```python
from build123d import *

# Parameters (mm, degrees)
BASE_DEPTH          = 3
SKETCH2_R           = 1.5
CUT_EXTRUDE1_DEPTH  = 36.920050111
CUT_EXTRUDE2_DEPTH  = 36.920050111
SKETCH6_R           = 3
CUT_EXTRUDE3_DEPTH  = 1.5
CHAMFER2_SIZE       = 0.5
BOSS_EXTRUDE1_START = -2.5
BOSS_EXTRUDE1_DEPTH = 2.5
CUT_EXTRUDE4_START  = -2.5
CUT_EXTRUDE4_DEPTH  = 2.5


# Read off the part's stored shape, not the designer's step: Cut-Extrude4
with BuildPart() as part:
    # Sketch1 → Base (new body)
    with BuildSketch(Plane.XY):
        with BuildLine():
            Line((11, -32.5), (-11, -32.5))
            ThreePointArc((-11, -32.5), (-13.828427125, -31.328427125), (-15, -28.5))
            Line((-15, -28.5), (-15, 28.5))
            ThreePointArc((-15, 28.5), (-13.828427125, 31.328427125), (-11, 32.5))
            Line((-11, 32.5), (11, 32.5))
            ThreePointArc((11, 32.5), (13.828427125, 31.328427125), (15, 28.5))
            Line((15, 28.5), (15, -28.5))
            ThreePointArc((15, -28.5), (13.828427125, -31.328427125), (11, -32.5))
        make_face()
    extrude(amount=BASE_DEPTH)

    # Sketch2 → Cut-Extrude1 (cut, through all)
    with BuildSketch(Plane.XY.offset(3)):
        with Locations((-11, 28.5)):
            Circle(SKETCH2_R)
        with Locations((-11, -28.5)):
            Circle(SKETCH2_R)
        with Locations((11, -28.5)):
            Circle(SKETCH2_R)
        with Locations((11, 28.5)):
            Circle(SKETCH2_R)
    extrude(amount=-CUT_EXTRUDE1_DEPTH, mode=Mode.SUBTRACT)

    # Sketch3 → Cut-Extrude2 (cut, through all)
    with BuildSketch(Plane.XY.offset(3)):
        with BuildLine():
            Line((6.5, 28.5), (6.5, 30.5))
            Line((6.5, 30.5), (-6.5, 30.5))
            Line((-6.5, 30.5), (-6.5, 28.5))
            ThreePointArc((-6.5, 28.5), (-7.818019485, 25.318019485), (-11, 24))
            Line((-11, 24), (-13, 24))
            Line((-13, 24), (-13, -24))
            Line((-13, -24), (-11, -24))
            ThreePointArc((-11, -24), (-7.818019485, -25.318019485), (-6.5, -28.5))
            Line((-6.5, -28.5), (-6.5, -30.5))
            Line((-6.5, -30.5), (6.5, -30.5))
            Line((6.5, -30.5), (6.5, -28.5))
            ThreePointArc((6.5, -28.5), (7.818019485, -25.318019485), (11, -24))
            Line((11, -24), (13, -24))
            Line((13, -24), (13, 24))
            Line((13, 24), (11, 24))
            ThreePointArc((11, 24), (7.818019485, 25.318019485), (6.5, 28.5))
        make_face()
    extrude(amount=-CUT_EXTRUDE2_DEPTH, mode=Mode.SUBTRACT)

    # Sketch6 → Cut-Extrude3 (cut)
    with BuildSketch(Plane.XY.offset(3)):
        with Locations((-11, -28.5)):
            Circle(SKETCH6_R)
        with Locations((11, -28.5)):
            Circle(SKETCH6_R)
        with Locations((11, 28.5)):
            Circle(SKETCH6_R)
        with Locations((-11, 28.5)):
            Circle(SKETCH6_R)
    extrude(amount=-CUT_EXTRUDE3_DEPTH, mode=Mode.SUBTRACT)

    # Chamfer2
    chamfer2_edges = [part.edges().sort_by_distance(p)[0] for p in [
        (7.818019485, 25.318019485, 3),
        (13, 0, 3),
        (7.818019485, -25.318019485, 3),
        (-7.818019485, -25.318019485, 3),
        (-13, 0, 3),
        (-7.818019485, 25.318019485, 3),
        (0, -32.5, 3),
        (-13.828427125, -31.328427125, 3),
        (-15, 0, 3),
        (-13.828427125, 31.328427125, 3),
        (0, 32.5, 3),
        (13.828427125, 31.328427125, 3),
        (15, 0, 3),
        (13.828427125, -31.328427125, 3),
        (-14, -28.5, 3),
        (-14, 28.5, 3),
        (8, 28.5, 3),
        (8, -28.5, 3),
        (0, -30.5, 3),
        (0, 30.5, 3),
        (12, 24, 3),
        (6.5, 29.5, 3),
        (-6.5, 29.5, 3),
        (-12, 24, 3),
        (-12, -24, 3),
        (-6.5, -29.5, 3),
        (6.5, -29.5, 3),
        (12, -24, 3),
    ]]
    chamfer(chamfer2_edges, length=CHAMFER2_SIZE - 0.0001)  # a hair under: the kernel refuses the full size

    # Sketch9 → Boss-Extrude1 (add)
    with BuildSketch(Plane(origin=(0, 0, 0), x_dir=(-1, 0, 0), z_dir=(0, 0, -1)).offset(BOSS_EXTRUDE1_START)):
        with BuildLine():
            ThreePointArc((-6.5, -28.5), (-7.818019485, -25.318019485), (-11, -24))
            Line((-11, -24), (-13, -24))
            Line((-13, -24), (-13, 24))
            Line((-13, 24), (-11, 24))
            ThreePointArc((-11, 24), (-7.818019485, 25.318019485), (-6.5, 28.5))
            Line((-6.5, 28.5), (-6.5, 30.5))
            Line((-6.5, 30.5), (6.5, 30.5))
            Line((6.5, 30.5), (6.5, 28.5))
            ThreePointArc((6.5, 28.5), (7.818019485, 25.318019485), (11, 24))
            Line((11, 24), (13, 24))
            Line((13, 24), (13, -24))
            Line((13, -24), (11, -24))
            ThreePointArc((11, -24), (7.818019485, -25.318019485), (6.5, -28.5))
            Line((6.5, -28.5), (6.5, -30.5))
            Line((6.5, -30.5), (-6.5, -30.5))
            Line((-6.5, -30.5), (-6.5, -28.5))
        make_face()
    extrude(amount=BOSS_EXTRUDE1_DEPTH)

    # Cut-Extrude4 outline → Cut-Extrude4 (cut)
    with BuildSketch(Plane(origin=(0, 0, 0), x_dir=(-1, 0, 0), z_dir=(0, 0, -1)).offset(CUT_EXTRUDE4_START)):
        with BuildLine():
            ThreePointArc((11.25, -6.35), (12.75, -4.85), (11.25, -3.35))
            Line((11.25, -3.35), (-11.25, -3.35))
            ThreePointArc((-11.25, -3.35), (-12.75, -4.85), (-11.25, -6.35))
            Line((-11.25, -6.35), (11.25, -6.35))
        make_face()
        with BuildLine():
            ThreePointArc((11.25, 17.9), (12.75, 19.4), (11.25, 20.9))
            Line((11.25, 20.9), (-11.25, 20.9))
            ThreePointArc((-11.25, 20.9), (-12.75, 19.4), (-11.25, 17.9))
            Line((-11.25, 17.9), (11.25, 17.9))
        make_face()
        with BuildLine():
            Line((-11, 24), (-12.729019946, 24))
            ThreePointArc((-12.729019946, 24), (-12.218245837, 23.104356076), (-11.25, 22.75))
            Line((-11.25, 22.75), (11.25, 22.75))
            ThreePointArc((11.25, 22.75), (12.218245837, 23.104356076), (12.729019946, 24))
            Line((12.729019946, 24), (11, 24))
            ThreePointArc((11, 24), (9.015686517, 24.461126395), (7.438048288, 25.75))
            Line((7.438048288, 25.75), (-7.438048288, 25.75))
            ThreePointArc((-7.438048288, 25.75), (-9.015686517, 24.461126395), (-11, 24))
        make_face()
        with BuildLine():
            ThreePointArc((-6.5, 28.5), (-6.522787311, 28.047709671), (-6.590918463, 27.6))
            Line((-6.590918463, 27.6), (6.590918463, 27.6))
            ThreePointArc((6.590918463, 27.6), (6.522787311, 28.047709671), (6.5, 28.5))
            Line((6.5, 28.5), (6.5, 30.5))
            Line((6.5, 30.5), (-6.5, 30.5))
            Line((-6.5, 30.5), (-6.5, 28.5))
        make_face()
        with BuildLine():
            Line((-6.5, -28.5), (-6.5, -30.5))
            Line((-6.5, -30.5), (6.5, -30.5))
            Line((6.5, -30.5), (6.5, -28.5))
            ThreePointArc((6.5, -28.5), (6.522787311, -28.047709671), (6.590918463, -27.6))
            Line((6.590918463, -27.6), (-6.590918463, -27.6))
            ThreePointArc((-6.590918463, -27.6), (-6.522787311, -28.047709671), (-6.5, -28.5))
        make_face()
        with BuildLine():
            Line((-11.25, -1.5), (11.25, -1.5))
            ThreePointArc((11.25, -1.5), (12.75, 0), (11.25, 1.5))
            Line((11.25, 1.5), (-11.25, 1.5))
            ThreePointArc((-11.25, 1.5), (-12.75, 0), (-11.25, -1.5))
        make_face()
        with BuildLine():
            ThreePointArc((11.25, -11.2), (12.75, -9.7), (11.25, -8.2))
            Line((11.25, -8.2), (-11.25, -8.2))
            ThreePointArc((-11.25, -8.2), (-12.75, -9.7), (-11.25, -11.2))
            Line((-11.25, -11.2), (11.25, -11.2))
        make_face()
        with BuildLine():
            ThreePointArc((11.25, -16.05), (12.75, -14.55), (11.25, -13.05))
            Line((11.25, -13.05), (-11.25, -13.05))
            ThreePointArc((-11.25, -13.05), (-12.75, -14.55), (-11.25, -16.05))
            Line((-11.25, -16.05), (11.25, -16.05))
        make_face()
        with BuildLine():
            ThreePointArc((11.25, -20.9), (12.75, -19.4), (11.25, -17.9))
            Line((11.25, -17.9), (-11.25, -17.9))
            ThreePointArc((-11.25, -17.9), (-12.75, -19.4), (-11.25, -20.9))
            Line((-11.25, -20.9), (11.25, -20.9))
        make_face()
        with BuildLine():
            ThreePointArc((12.729019946, -24), (12.218245837, -23.104356076), (11.25, -22.75))
            Line((11.25, -22.75), (-11.25, -22.75))
            ThreePointArc((-11.25, -22.75), (-12.218245837, -23.104356076), (-12.729019946, -24))
            Line((-12.729019946, -24), (-11, -24))
            ThreePointArc((-11, -24), (-9.015686517, -24.461126395), (-7.438048288, -25.75))
            Line((-7.438048288, -25.75), (7.438048288, -25.75))
            ThreePointArc((7.438048288, -25.75), (9.015686517, -24.461126395), (11, -24))
            Line((11, -24), (12.729019946, -24))
        make_face()
        with BuildLine():
            ThreePointArc((11.25, 3.35), (12.75, 4.85), (11.25, 6.35))
            Line((11.25, 6.35), (-11.25, 6.35))
            ThreePointArc((-11.25, 6.35), (-12.75, 4.85), (-11.25, 3.35))
            Line((-11.25, 3.35), (11.25, 3.35))
        make_face()
        with BuildLine():
            ThreePointArc((11.25, 8.2), (12.75, 9.7), (11.25, 11.2))
            Line((11.25, 11.2), (-11.25, 11.2))
            ThreePointArc((-11.25, 11.2), (-12.75, 9.7), (-11.25, 8.2))
            Line((-11.25, 8.2), (11.25, 8.2))
        make_face()
        with BuildLine():
            ThreePointArc((11.25, 13.05), (12.75, 14.55), (11.25, 16.05))
            Line((11.25, 16.05), (-11.25, 16.05))
            ThreePointArc((-11.25, 16.05), (-12.75, 14.55), (-11.25, 13.05))
            Line((-11.25, 13.05), (11.25, 13.05))
        make_face()
    extrude(amount=CUT_EXTRUDE4_DEPTH, mode=Mode.SUBTRACT)


solid = part.part
```
Geometry check sheet. Reference: the model listing, model coordinates, mm. A direction names the side the tool comes from. Give positions to 0.01 mm unless a question says otherwise; leave off trailing zeros. Order: outer loops, then holes, each group sorted by start corner. A loop starts at its lowest first (then second) coordinate and runs counter-clockwise, first axis right, second up. Notation, with made-up numbers: (-30, 86) - (12, 86) arc R7 ccw to (12, 91) - close; hole circle Ø5 at (-23, 6). An arc over 180 degrees is marked (long way). Write item = value, one per line. Start each with the question number.
1) Draft check along Y on faces 1 (the cylindrical face through (11, 30, 1)), 2 (the flat face through (-15, 0, 1)), 3 (the flat face through (0, -1.5, 1)), 4 (the cylindrical face through (-13.859, 31.297, 1.233)). Enter one of: released by +Y, released by -Y, zero draft, split by the parting line, or undercut.
2) Section check C-C (z = 1). Count the separate pieces of the cut face and the enclosed holes in it, then the cut area to 3 significant figures.
3) Access from +Z, -Z, +X, -X, +Y, -Y to the whole of each face (thin tool, end or side, straight path). Record for faces 5 (the conical face through (-8.039, 25.603, 2.858)), 6 (the flat face through (0, 1.5, 1)), 7 (the flat face through (0, -32.5, 1)).
4) Section check B-B (y = 7). Enter the section's corners in (x, z).
5) Gauge pin test, flat ends, axial feed: pin 1 Ø3.5 at (x, y) = (11, -28.5) entering from +Z; pin 2 Ø3 at (x, y) = (5, 3) entering from -Z; pin 3 Ø4 at (x, y) = (-10.5, -20) entering from +Z; pin 4 Ø1.6 at (x, z) = (-12.5, 1.5) entering from +Y. Record the tip position at first contact, or that the pin passes through.
6) Scan lines: L1, parallel to X at y = 28, z = 0.9; L2, parallel to Z at x = -7.25, y = -26; L3, parallel to X at y = -28, z = 1.55. Record each from-to range of solid material in increasing order.
7) Section check A-A (y = 19.4). Enter the section's corners in (x, z).
Geometry check:
q1.face_1 = undercut
q1.face_2 = zero draft
q1.face_3 = undercut
q1.face_4 = released by +Y
q2.separate_pieces = 1
q2.enclosed_holes = 17
q2.area = 1,040 mm2
q3.face_5 = +Z
q3.face_6 = +Z, -Z
q3.face_7 = +Z, -Z, +X, -X, -Y
q4.outline = (-15, 0) - (15, 0) - (15, 2.5) - (14.5, 3) - (13.5, 3) - (13, 2.5) - (-13, 2.5) - (-13.5, 3) - (-14.5, 3) - (-15, 2.5) - close
q5.pin_1 = 1.5
q5.pin_2 = 0
q5.pin_3 = 2.5
q5.pin_4 = 32.44
q6.L1 = -15 to -12.41, -9.59 to -6.53, 6.53 to 9.59, 12.41 to 15
q6.L2 = 0 to 2.5
q6.L3 = -15 to -13.96, -8.04 to -6.53, 6.53 to 8.04, 13.96 to 15
q7.outline = (-15, 0) - (-12.75, 0) - (-12.75, 2.5) - (-13, 2.5) - (-13.5, 3) - (-14.5, 3) - (-15, 2.5) - close; (12.75, 0) - (15, 0) - (15, 2.5) - (14.5, 3) - (13.5, 3) - (13, 2.5) - (12.75, 2.5) - close
